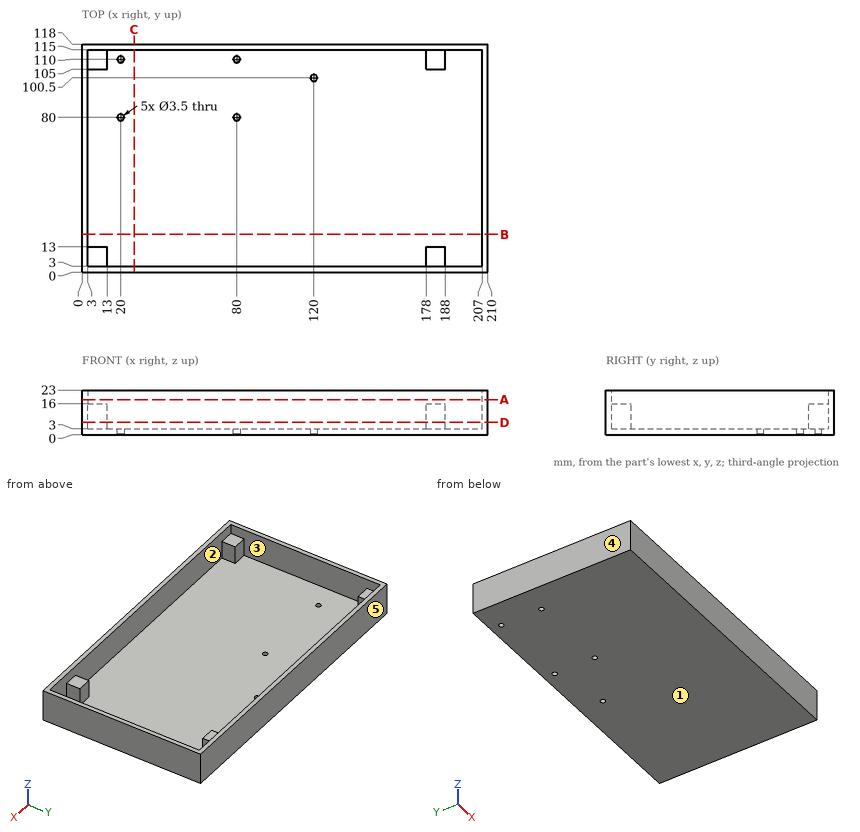
Here's the drawing with two shaded views (mm, measured from the low corner). I have some questions. A direction names the side the tool comes from. Round coordinates to 2 decimals unless told otherwise and drop trailing zeros. Loops run counter-clockwise (first coordinate to the right, second up) from the corner with the lowest first, then second, coordinate; pieces in that order, holes last. Notation, with made-up numbers: M -30,71 L -6,71 A21 ccw -6,103 Z; hole C -29,-5 d10. An arc over 180 degrees is marked long. Answer as a JSON object with one key per item and string values. Group by question number.
Q1. Imagine slicing it at D-D, the plane z = 6.25. Please give me the cut outline in (x, y), then the cut area to 3 significant figures.
Q2. Imagine slicing it at A-A, the plane z = 18. Please give me the cut outline in (x, y).
Q3. On a 3-axis mill with a long thin cutter (end or side, diameter ignored), from which of +Z, -Z, +X, -X, +Y, -Y can I reach the whole of each face in a straight line? I mean the marked faces 1 and 2. Say none if no direction works.
Q4. Please list where these lines run through material, in increasing order: L1, parallel to X at y = 80, z = 1.15; L2, parallel to Y at x = 20, z = 1.95; L3, parallel to X at y = 81.5, z = 15.
Q5. Imagine slicing it at B-B, the plane y = 19.5. Please give me the cut outline in (x, z), then the cut area to 3 significant figures.
Q6. Will these pins go through, and if not, where does the flat tip stop? pin 1 (3 mm diameter, centred on x = 80, y = 110, fed in from -Z); pin 2 (5 mm diameter, centred on x = 80, y = 104.5, fed in from +Z); pin 3 (3 mm diameter, centred on x = 6.5, y = 10, fed in from +Z).
Q7. We'd pull the mould along Y, two halves only. Please class the marked faces 3, 4 and 5: +Y half, -Y half, draft (parallel to the pull), parting line (faces both ways), or undercut.
Q8. Imagine slicing it at C-C, the plane x = 27. Please give me the cut outline in (y, z).
Findings:
{
 "1": {"outline": "M 0,0 L 210,0 L 210,118 L 0,118 Z; hole M 3,13 L 13,13 L 13,3 L 178,3 L 178,13 L 188,13 L 188,3 L 207,3 L 207,115 L 188,115 L 188,105 L 178,105 L 178,115 L 13,115 L 13,105 L 3,105 Z", "area": "2,330 mm2"},
 "2": {"outline": "M 0,0 L 210,0 L 210,118 L 0,118 Z; hole M 3,3 L 207,3 L 207,115 L 3,115 Z"},
 "3": {"face 1": "-Z, +X, -X, +Y, -Y", "face 2": "+Z"},
 "4": {"L1": "x = 0 to 18.25, 21.75 to 78.25, 81.75 to 210", "L2": "y = 0 to 78.25, 81.75 to 108.25, 111.75 to 118", "L3": "x = 0 to 3, 207 to 210"},
 "5": {"outline": "M 0,0 L 210,0 L 210,23 L 207,23 L 207,3 L 3,3 L 3,23 L 0,23 Z", "area": "750 mm2"},
 "6": {"pin 1": "passes through", "pin 2": "stops at z = 3", "pin 3": "stops at z = 16"},
 "7": {"face 3": "undercut", "face 4": "draft", "face 5": "+Y half"},
 "8": {"outline": "M 0,0 L 118,0 L 118,23 L 115,23 L 115,3 L 3,3 L 3,23 L 0,23 Z"}
}
